For this review, take the finished solid that the model builds, in its own axes (mm). A direction names the side the tool comes from. Give positions to 0.01 mm unless a question says otherwise; leave off trailing zeros. Write each loop counter-clockwise with the first axis right and the second up, starting at its lowest first coordinate (ties: lowest second). Pieces come first, ordered by that corner, then holes. Notation, with made-up numbers: (45.25, -11) -> (61.25, -11) arc R4 ccw to (61.25, -5) -> close; hole circle Ø11 at (32, -30.75). An arc over 180 degrees is marked (long way). Return JSON: item names as keys, results as strings.
from build123d import *

# Parameters (mm, degrees)
SKETCH1_R                                = 15.875
BOSS_EXTRUDE1_DEPTH                      = 3.81
SKETCH2_R                                = 5.715
CUT_EXTRUDE1_DEPTH                       = 23.771634768
SKETCH3_R                                = 6.35
CUT_EXTRUDE3_DEPTH                       = 1.27
F_1_16_0_0625_DIAMETER_HOLE1_D           = 1.5875
F_1_16_0_0625_DIAMETER_HOLE1_CSINK_D     = 2.8575
F_1_16_0_0625_DIAMETER_HOLE1_CSINK_ANGLE = 100
CIRPATTERN1_COUNT                        = 3


with BuildPart() as part:
    # Sketch1 → Boss-Extrude1 (new body)
    with BuildSketch(Plane.XY):
        with Locations(Location((0, 0, 0), (0, 0, 180))):
            Circle(SKETCH1_R)
    extrude(amount=BOSS_EXTRUDE1_DEPTH)

    # Sketch2 → Cut-Extrude1 (cut, through all)
    with BuildSketch(Plane.XY.offset(3.81)):
        Circle(SKETCH2_R)
    extrude(amount=-CUT_EXTRUDE1_DEPTH, mode=Mode.SUBTRACT)

    # Sketch3 → Cut-Extrude3 (cut)
    with BuildSketch(Plane(origin=(0, 0, 0), x_dir=(-1, 0, 0), z_dir=(0, 0, -1))):
        Circle(SKETCH3_R)
    extrude(amount=-CUT_EXTRUDE3_DEPTH, mode=Mode.SUBTRACT)

    # 1/16 (0.0625) Diameter Hole1 (through all)
    with Locations(Plane.XY.offset(3.81)):
        with Locations((7.60482237, 8.532969982)):
            f_1_16_0_0625_diameter_hole1 = CounterSinkHole(F_1_16_0_0625_DIAMETER_HOLE1_D / 2, F_1_16_0_0625_DIAMETER_HOLE1_CSINK_D / 2, counter_sink_angle=F_1_16_0_0625_DIAMETER_HOLE1_CSINK_ANGLE)

    # CirPattern1: 1/16 (0.0625) Diameter Hole1 ×3 about axis
    cirpattern1_axis = Axis((0, 0, 0), (0, 0, 1))
    for i in range(1, CIRPATTERN1_COUNT):
        add(f_1_16_0_0625_diameter_hole1.rotate(cirpattern1_axis, i * 360 / CIRPATTERN1_COUNT), mode=Mode.SUBTRACT)


solid = part.part
1. Add section D-D, the plane x = 11. State the section outline as (y, z) points, plus the area to 3 significant figures.
Results found:
{"outline": "(-11.45, 0) -> (11.45, 0) -> (11.45, 3.81) -> (-11.45, 3.81) -> close", "area": "87.2 mm²"}
2. Add section A-A, the plane x = 0. State the section outline as (y, z) points (3 decimals).
Results found:
{"outline": "(-15.875, 0) -> (-6.35, 0) -> (-6.35, 1.27) -> (-5.715, 1.27) -> (-5.715, 3.81) -> (-15.875, 3.81) -> close; (5.715, 1.27) -> (6.35, 1.27) -> (6.35, 0) -> (15.875, 0) -> (15.875, 3.81) -> (5.715, 3.81) -> close"}
3. Add section C-C, the plane z = 0.8. Count the separate pieces of the cut face and the enclosed holes in it, plus the area to 3 significant figures.
Results found:
{"separate pieces": "1", "enclosed holes": "4", "area": "659 mm²"}
4. The part is to be moulded in two halves that separate along Y. For faces 3 (the cylindrical face through (6.848, 8.771, 1.616)), 4 (the cylindrical face through (5.45, 1.72, 2.56)), 5 (the flat face through (0, 7, 0)), 6 (the cylindrical face through (3.441, 15.497, 1.878)), say which applies: +Y half, -Y half, draft (parallel to the pull), parting line (faces both ways), or undercut.
Results found:
{"face 3": "undercut", "face 4": "undercut", "face 5": "draft", "face 6": "parting line"}
5. For pin 1 (2 mm diameter, centred on y = -5, z = 1.5, fed in from +X); pin 2 (1.8 mm diameter, centred on x = 7.6, y = 8.53, fed in from +Z); pin 3 (10 mm diameter, centred on x = 0.5, y = 1, fed in from -Z), all flat-tipped, find the tip position at first contact; note any pin that passes through.
Results found:
{"pin 1": "stops at x = 15.36", "pin 2": "stops at z = 3.37", "pin 3": "stops at z = 1.27"}
6. For faces 1 (the flat face through (0, 7, 3.81)), 2 (the cylindrical face through (1.38, -6.2, 0.63)), list the 3-axis set-ups (+Z, -Z, +X, -X, +Y, -Y) from which the entire face can be reached by the end or side of a thin tool; tool diameter is ignored.
Results found:
{"face 1": "+Z, +X, -X, +Y, -Y", "face 2": "-Z"}
7. To check wall thickness, follow probe 1 along Y at (x, z) = (0, 2.8) (3 decimals); probe 2 along Y at (x, z) = (3.5, 1.5); probe 3 along X at (y, z) = (3, 2.9). State the ranges of each line that lie inside material, in increasing order.
Results found:
{"probe 1": "y = -15.875 to -5.715, 5.715 to 15.875", "probe 2": "y = -15.48 to -11.64, -10.06 to -4.52, 4.52 to 15.48", "probe 3": "x = -15.59 to -11.6, -10.78 to -4.86, 4.86 to 15.59"}
